Check sheet for the modelled part. Datum: model origin and axes. Units: mm. A direction names the side the tool comes from. Give positions to 0.01 mm unless a question says otherwise; leave off trailing zeros. Loops run counter-clockwise (first coordinate to the right, second up) from the corner with the lowest first, then second, coordinate; pieces in that order, holes last. Notation, with made-up numbers: (75, -27.75) - (112, -27.75) arc R24 ccw to (112, -11.75) - close; hole circle Ø4 at (57, 21). An arc over 180 degrees is marked (long way). Answer in a Markdown table with one row per item. Add a question column.
(1) Sectioned sample at A-A on z = -28. Enter the section's corners in (x, y), then the cut area to 3 significant figures.
(2) Sectioned sample at D-D on z = 15. Enter the section's corners in (x, y), then the cut area to 3 significant figures.
(3) Draft check along Z on faces 1 (the face through (-56.99, -54.79, -42.15)), 2 (the face through (-3, 2, 20)), 3 (the face through (-72.15, -54.93, -56.99)), 4 (the face through (96.92, -118.31, 12.4)). Enter one of: released by +Z, released by -Z, zero draft, split by the parting line, or undercut.
(4) Sectioned sample at C-C on y = -105. Enter the section's corners in (x, z).
(5) Set-up check for faces 5 (the face through (0, -70, -47)), 6 (the face through (-1, -55, -45)), 7 (the face through (75, -55, -27)): record each of +Z, -Z, +X, -X, +Y, -Y from which the full face is reachable in a straight line by a thin tool's end or side.
(6) Sectioned sample at B-B on x = -90. Enter the section's corners in (y, z), then the cut area to 3 significant figures.
(7) Thickness scan on L1, parallel to Y at x = 90, z = 10.75; L2, parallel to Z at x = -90, y = -85; L3, parallel to X at y = -102, z = 5. Record the ranges inside material, lowest first.
(8) Go/stop test with flat-tipped pins: P1, Ø5, axis at x = 73.5, y = -90.5, coming from the -Z side; P2, Ø24, axis at y = -58.5, z = -22.5, coming from the -X side; P3, Ø5, axis at y = -56.5, z = -30, coming from the +X side. Record where each tip stops, or that it passes through.
from build123d import *

# Parameters (mm, degrees)
SCHIZZO1_W                   = 360
SCHIZZO1_H                   = 280
SCHIZZO1_R                   = 15
ESTRUSIONE_ESTRUSIONE1_DEPTH = 20
SCHIZZO2_W                   = 150
SCHIZZO2_H                   = 30
ESTRUSIONE_ESTRUSIONE2_DEPTH = 60
SCHIZZO3_W                   = 120
SCHIZZO3_H                   = 45
TAGLIO_ESTRUSIONE2_DEPTH     = 30
RACCORDO2_R                  = 10
RACCORDO3_R                  = 10
RACCORDO4_R                  = 10
RACCORDO5_R                  = 10
RACCORDO6_R                  = 10
RACCORDO7_R                  = 10
RACCORDO8_R                  = 10
RACCORDO12_R                 = 5


with BuildPart() as part:
    # Schizzo1 → Estrusione-Estrusione1 (new body)
    with BuildSketch(Plane.XY):
        Rectangle(SCHIZZO1_W, SCHIZZO1_H)
        with Locations((-90, -105)):
            Circle(SCHIZZO1_R, mode=Mode.SUBTRACT)
        with Locations((90, -105)):
            Circle(SCHIZZO1_R, mode=Mode.SUBTRACT)
        with Locations((0, -105)):
            Circle(SCHIZZO1_R, mode=Mode.SUBTRACT)
    extrude(amount=ESTRUSIONE_ESTRUSIONE1_DEPTH)

    # Schizzo2 → Estrusione-Estrusione2 (add)
    with BuildSketch(Plane(origin=(0, 0, 0), x_dir=(-1, 0, 0), z_dir=(0, 0, -1))):
        with Locations((0, -55)):
            Rectangle(SCHIZZO2_W, SCHIZZO2_H)
    extrude(amount=ESTRUSIONE_ESTRUSIONE2_DEPTH)

    # Schizzo3 → Taglio-Estrusione2 (cut)
    with BuildSketch(Plane.XZ.offset(70)):
        with Locations((0, -22.5)):
            Rectangle(SCHIZZO3_W, SCHIZZO3_H)
    extrude(amount=-TAGLIO_ESTRUSIONE2_DEPTH, mode=Mode.SUBTRACT)

    # Raccordo2
    raccordo2_edges = [part.edges().sort_by_distance(p)[0] for p in [
        (-75, -55, -60),
        (0, -40, -60),
        (75, -55, -60),
        (0, -70, -60),
    ]]
    fillet(raccordo2_edges, radius=RACCORDO2_R)

    # Raccordo3
    raccordo3_edges = [part.edges().sort_by_distance(p)[0] for p in [
        (60, -55, -45),
    ]]
    fillet(raccordo3_edges, radius=RACCORDO3_R)

    # Raccordo4
    raccordo4_edges = [part.edges().sort_by_distance(p)[0] for p in [
        (-60, -55, -45),
    ]]
    fillet(raccordo4_edges, radius=RACCORDO4_R)

    # Raccordo5
    # the kernel refuses this fillet: 10 mm, written as the material it takes off along each edge
    with BuildSketch(Plane(origin=(65, -60, -50), x_dir=(1, 0, 0), z_dir=(0, -1, 0))) as raccordo5_piece_1_section:
        Polygon((0, 0), (RACCORDO5_R, 0), (RACCORDO5_R, -RACCORDO5_R), (0, -RACCORDO5_R), align=None)
    raccordo5_piece_1 = extrude(amount=RACCORDO5_R, mode=Mode.PRIVATE)
    raccordo5_piece_1 = raccordo5_piece_1 - Plane(origin=(65, -60, -50), x_dir=(-0.7071067811865475, 0, 0.7071067811865475), z_dir=(0, -1, 0)) * Sphere(RACCORDO5_R, mode=Mode.PRIVATE)
    add(raccordo5_piece_1, mode=Mode.SUBTRACT)
    with BuildSketch(Plane(origin=(75, -70, 0), x_dir=(-1, 0, 0), z_dir=(0, 0, -1))) as raccordo5_piece_2:
        with BuildLine():
            CenterArc((RACCORDO5_R, RACCORDO5_R), RACCORDO5_R, 180, 90)
            Line((0, RACCORDO5_R), (0, 0))
            Line((0, 0), (RACCORDO5_R, 0))
        make_face()
    extrude(amount=50, mode=Mode.SUBTRACT)

    # Raccordo6
    # the kernel refuses this fillet: 10 mm, written as the material it takes off along each edge
    with BuildSketch(Plane(origin=(-65, -50, -50), x_dir=(0, 1, 0), z_dir=(-1, 0, 0))) as raccordo6_piece_1_section:
        Polygon((0, 0), (RACCORDO6_R, 0), (RACCORDO6_R, RACCORDO6_R), (0, RACCORDO6_R), align=None)
    raccordo6_piece_1 = extrude(amount=RACCORDO6_R, mode=Mode.PRIVATE)
    raccordo6_piece_1 = raccordo6_piece_1 - Plane(origin=(-65, -50, -50), x_dir=(0, -0.7071067811865475, 0.7071067811865475), z_dir=(-1, 0, 0)) * Sphere(RACCORDO6_R, mode=Mode.PRIVATE)
    add(raccordo6_piece_1, mode=Mode.SUBTRACT)
    with BuildSketch(Plane(origin=(-75, -40, 0), x_dir=(0, -1, 0), z_dir=(0, 0, -1))) as raccordo6_piece_2:
        with BuildLine():
            CenterArc((RACCORDO6_R, -RACCORDO6_R), RACCORDO6_R, 90, 90)
            Line((0, -RACCORDO6_R), (0, 0))
            Line((0, 0), (RACCORDO6_R, 0))
        make_face()
    extrude(amount=50, mode=Mode.SUBTRACT)

    # Raccordo7
    # the kernel refuses this fillet: 10 mm, written as the material it takes off along each edge
    with BuildSketch(Plane(origin=(65, -50, -50), x_dir=(1, 0, 0), z_dir=(0, 1, 0))) as raccordo7_piece_1_section:
        Polygon((0, 0), (RACCORDO7_R, 0), (RACCORDO7_R, RACCORDO7_R), (0, RACCORDO7_R), align=None)
    raccordo7_piece_1 = extrude(amount=RACCORDO7_R, mode=Mode.PRIVATE)
    raccordo7_piece_1 = raccordo7_piece_1 - Plane(origin=(65, -50, -50), x_dir=(-0.7071067811865475, 0, 0.7071067811865475), z_dir=(0, 1, 0)) * Sphere(RACCORDO7_R, mode=Mode.PRIVATE)
    add(raccordo7_piece_1, mode=Mode.SUBTRACT)
    with BuildSketch(Plane(origin=(75, -40, 0), x_dir=(-1, 0, 0), z_dir=(0, 0, -1))) as raccordo7_piece_2:
        with BuildLine():
            CenterArc((RACCORDO7_R, -RACCORDO7_R), RACCORDO7_R, 90, 90)
            Line((0, -RACCORDO7_R), (0, 0))
            Line((0, 0), (RACCORDO7_R, 0))
        make_face()
    extrude(amount=50, mode=Mode.SUBTRACT)

    # Raccordo8
    # the kernel refuses this fillet: 10 mm, written as the material it takes off along each edge
    with BuildSketch(Plane(origin=(-65, -60, -50), x_dir=(-1, 0, 0), z_dir=(0, -1, 0))) as raccordo8_piece_1_section:
        Polygon((0, 0), (RACCORDO8_R, 0), (RACCORDO8_R, RACCORDO8_R), (0, RACCORDO8_R), align=None)
    raccordo8_piece_1 = extrude(amount=RACCORDO8_R, mode=Mode.PRIVATE)
    raccordo8_piece_1 = raccordo8_piece_1 - Plane(origin=(-65, -60, -50), x_dir=(0.7071067811865475, 0, 0.7071067811865475), z_dir=(0, -1, 0)) * Sphere(RACCORDO8_R, mode=Mode.PRIVATE)
    add(raccordo8_piece_1, mode=Mode.SUBTRACT)
    with BuildSketch(Plane(origin=(-75, -70, 0), x_dir=(1, 0, 0), z_dir=(0, 0, -1))) as raccordo8_piece_2:
        with BuildLine():
            CenterArc((RACCORDO8_R, -RACCORDO8_R), RACCORDO8_R, 90, 90)
            Line((0, -RACCORDO8_R), (0, 0))
            Line((0, 0), (RACCORDO8_R, 0))
        make_face()
    extrude(amount=50, mode=Mode.SUBTRACT)

    # Raccordo12
    raccordo12_edges = [part.edges().sort_by_distance(p)[0] for p in [
        (72.071067812, -67.071067812, 0),
        (-62.5, -40, 0),
        (-72.071067812, -42.928932188, 0),
        (75, -55, 0),
        (72.071067812, -42.928932188, 0),
        (-105, -105, 0),
        (-75, -55, 0),
        (-72.071067812, -67.071067812, 0),
        (75, -105, 0),
        (-15, -105, 0),
        (-62.5, -70, 0),
        (62.5, -40, 0),
        (60, -55, 0),
        (-60, -55, 0),
        (0, -140, 0),
        (-180, 0, 0),
        (0, 140, 0),
        (180, 0, 0),
        (62.5, -70, 0),
    ]]
    fillet(raccordo12_edges, radius=RACCORDO12_R)


solid = part.part
Reply:
| question | item | result |
|---|---|---|
| 1 | outline | (-75, -60) arc R10 ccw to (-65, -70) - (-60, -70) - (-60, -40) - (-65, -40) arc R10 ccw to (-75, -50) - close; (60, -70) - (65, -70) arc R10 ccw to (75, -60) - (75, -50) arc R10 ccw to (65, -40) - (60, -40) - close |
| 1 | area | 814 mm^2 |
| 2 | outline | (-180, -140) - (180, -140) - (180, 140) - (-180, 140) - close; hole circle Ø30 at (-90, -105); hole circle Ø30 at (0, -105); hole circle Ø30 at (90, -105) |
| 2 | area | 98,700 mm^2 |
| 3 | face 1 | undercut |
| 3 | face 2 | released by +Z |
| 3 | face 3 | released by -Z |
| 3 | face 4 | zero draft |
| 4 | outline | (-180, 5) arc R5 ccw to (-175, 0) - (-110, 0) arc R5 ccw to (-105, 5) - (-105, 20) - (-180, 20) - close; (-75, 5) arc R5 ccw to (-70, 0) - (-20, 0) arc R5 ccw to (-15, 5) - (-15, 20) - (-75, 20) - close; (15, 5) arc R5 ccw to (20, 0) - (70, 0) arc R5 ccw to (75, 5) - (75, 20) - (15, 20) - close; (105, 5) arc R5 ccw to (110, 0) - (175, 0) arc R5 ccw to (180, 5) - (180, 20) - (105, 20) - close |
| 5 | face 5 | -Z, +X, -X, -Y |
| 5 | face 6 | +Y, -Y |
| 5 | face 7 | -Z, +X, +Y, -Y |
| 6 | outline | (-140, 5) arc R5 ccw to (-135, 0) - (-125, 0) arc R5 ccw to (-120, 5) - (-120, 20) - (-140, 20) - close; (-90, 5) arc R5 ccw to (-85, 0) - (135, 0) arc R5 ccw to (140, 5) - (140, 20) - (-90, 20) - close |
| 6 | area | 4,980 mm^2 |
| 7 | L1 | -140 to -120, -90 to 140 |
| 7 | L2 | 0 to 20 |
| 7 | L3 | -180 to -104.7, -75.3 to -14.7, 14.7 to 75.3, 104.7 to 180 |
| 8 | P1 | z = 0 |
| 8 | P2 | x = -75 |
| 8 | P3 | x = 75 |
